Verification items for the finished model (mm, model axes). A direction names the side the tool comes from. Coordinates: 2 decimals unless noted, no trailing zeros. Order: outer loops, then holes, each group sorted by start corner. A loop starts at its lowest first (then second) coordinate and runs counter-clockwise, first axis right, second up. Notation, with made-up numbers: (-27, 11) -> (11, 11) arc R14 ccw to (11, 25) -> close; hole circle Ø8 at (10.25, -26). An arc over 180 degrees is marked (long way). Answer as CSV lines item,"result".
```python
from build123d import *

# Parameters (mm, degrees)
SKETCH1_R           = 5
SKETCH1_R_2         = 2.5
BOSS_EXTRUDE1_DEPTH = 12
SKETCH2_R           = 1.75
BOSS_EXTRUDE2_DEPTH = 3.5


with BuildPart() as part:
    # Sketch1 → Boss-Extrude1 (new body)
    with BuildSketch(Plane(origin=(0, 0, 0), x_dir=(1, 0, 0), z_dir=(0, 1, 0))):
        Circle(SKETCH1_R)
        Circle(SKETCH1_R_2, mode=Mode.SUBTRACT)
    extrude(amount=BOSS_EXTRUDE1_DEPTH)

    # Sketch2 → Boss-Extrude2 (add)
    with BuildSketch(Plane(origin=(0, 0, 0), x_dir=(1, 0, 0), z_dir=(0, 1, 0))):
        with BuildLine():
            Line((0, -5), (-10.5, -5))
            ThreePointArc((-10.5, -5), (-12.5, 0), (-10.5, 5))
            Line((-10.5, 5), (0, 5))
            ThreePointArc((0, 5), (-5, 0), (0, -5))
        make_face()
        with Locations((-9, 0)):
            Circle(SKETCH2_R, mode=Mode.SUBTRACT)
    boss_extrude2 = extrude(amount=BOSS_EXTRUDE2_DEPTH)

    # Mirror1: Boss-Extrude2 across plane
    add(boss_extrude2.mirror(Plane(origin=(0, 0, 0), x_dir=(0, 0, 1), z_dir=(1, 0, 0))))


solid = part.part
```
Item 1: Section check C-C, the plane z = 0.5. Record the boundary of the cut face in (x, y).
Answer list:
outline,"(-12.48, 0) -> (-10.68, 0) -> (-10.68, 3.5) -> (-12.48, 3.5) -> close; (-7.32, 0) -> (-2.45, 0) -> (-2.45, 12) -> (-4.97, 12) -> (-4.97, 3.5) -> (-7.32, 3.5) -> close; (2.45, 0) -> (7.32, 0) -> (7.32, 3.5) -> (4.97, 3.5) -> (4.97, 12) -> (2.45, 12) -> close; (10.68, 0) -> (12.48, 0) -> (12.48, 3.5) -> (10.68, 3.5) -> close"
Item 2: Release check for a two-part mould opening along Z. For faces 1 (the cylindrical face through (7.331, 1.726, -0.526)), 2 (the cylindrical face through (-12.5, 1.7, 0.1)), 3 (the cylindrical face through (-7.331, 1.726, -0.526)), 4 (the flat face through (3, 0, 0)) record: +Z half, -Z half, draft (parallel to the pull), parting line (faces both ways), or undercut.
Answer list:
face 1,"undercut"
face 2,"parting line"
face 3,"undercut"
face 4,"draft"
Item 3: Section check A-A, the plane x = 9. Record the boundary of the cut face in (y, z).
Answer list:
outline,"(0, -5) -> (3.5, -5) -> (3.5, -1.75) -> (0, -1.75) -> close; (0, 1.75) -> (3.5, 1.75) -> (3.5, 5) -> (0, 5) -> close"
Item 4: Thickness scan on line 1 (X direction, y = 2, z = 0); line 2 (X direction, y = 8, z = 0); line 3 (Z direction, x = 9, y = 2.8). Record the ranges inside material, lowest first.
Answer list:
line 1,"-12.5 to -10.75, -7.25 to -2.5, 2.5 to 7.25, 10.75 to 12.5"
line 2,"-5 to -2.5, 2.5 to 5"
line 3,"-5 to -1.75, 1.75 to 5"
Item 5: Tool access check on faces 5 (the cylindrical face through (4.77, 7.69, -1.5)), 6 (the flat face through (0, 2, 5)). Record the directions out of +Z, -Z, +X, -X, +Y, -Y that give a thin tool (end or side, any length) a straight path to the whole face; none if there is none.
Answer list:
face 5,"+Y"
face 6,"+Z, +X, -X, +Y, -Y"
Item 6: Section check D-D, the plane y = 6. Record the boundary of the cut face in (x, z).
Answer list:
outline,"circle Ø10 at (0, 0); hole circle Ø5 at (0, 0)"
Item 7: Section check B-B, the plane y = 3. Record the boundary of the cut face in (x, z), plus the area to 3 significant figures.
Answer list:
outline,"(-10.5, -5) -> (10.5, -5) arc R7.25 ccw to (10.5, 5) -> (-10.5, 5) arc R7.25 ccw to start; hole circle Ø3.5 at (-9, 0); hole circle Ø5 at (0, 0); hole circle Ø3.5 at (9, 0)"
area,"199 mm2"
Item 8: Depth check by flat-ended pin: pin 1 Ø5 at (x, z) = (6, -0.5) entering from +Y; pin 2 Ø2 at (x, z) = (8.5, -1) entering from +Y; pin 3 Ø3 at (x, z) = (9, 0) entering from -Y. Enter the tip coordinate at first touch or a pass-through.
Answer list:
pin 1,"y = 12"
pin 2,"y = 3.5"
pin 3,"through"
